```python
from build123d import *

# Parameters (mm, degrees)
F1_DEPTH = 57
F2_DEPTH = 12


with BuildPart() as f1:
    # F0 (on Right) → F1 (new body)
    with BuildSketch(Plane.YZ):
        Polygon((1107.558378, 1620.736191), (1544.042206, 643.137381), (1586.458342, 548.137381), (1690.497414, 548.137381), (1132.390367, 1798.137381), (1064.487016, 1717.203709), align=None)
        Polygon((207.647976, 548.137381), (287.352976, 643.137381), (1107.558378, 1620.736191), (1064.487016, 1717.203709), (83.640367, 548.137381), align=None)
        Polygon((1586.458342, 548.137381), (1544.042206, 643.137381), (287.352976, 643.137381), (207.647976, 548.137381), align=None)
    extrude(amount=-F1_DEPTH)

    # F0 (on Right) → F2 (join)
    with BuildSketch(Plane.YZ):
        Polygon((287.352976, 643.137381), (1544.042206, 643.137381), (1107.558378, 1620.736191), align=None)
    extrude(amount=-F2_DEPTH)


solid = f1.part
```
Geometry: final body of the model. Coordinates: model frame, mm. A direction names the side the tool comes from. Round coordinates to 2 decimals unless told otherwise and drop trailing zeros. Write each loop counter-clockwise with the first axis right and the second up, starting at its lowest first coordinate (ties: lowest second). Pieces come first, ordered by that corner, then holes.
Item 1: Material intervals for L1, parallel to X at y = 1159, z = 869.5; L2, parallel to Y at x = -39.5, z = 964.5; L3, parallel to Y at x = -30.5, z = 651, sorted ascending.
Item 2: Mould query, pull axis Z, two halves, no side actions, for faces 1 (the face through (-28, 876, 548.137)), 2 (the face through (0, 876, 904)), 3 (the face through (-34.185, 1322.745, 1138.78)). Classes: +Z half, -Z half, draft (parallel to the pull), parting line (faces both ways), or undercut.
Item 3: Section query D-D (z = 1667). Return loops of the section in (x, y).
Item 4: Section query B-B (y = 595). Return loops of the section in (x, z), plus the area to 3 significant figures.
Item 5: Set-up query: faces 4 (the face through (-57, 705, 1176)), 5 (the face through (-12, 907, 922)). Return all of +Z, -Z, +X, -X, +Y, -Y with unobstructed straight access to the full face (end or side cutting, diameter ignored); none if empty.
Item 6: Section query C-C (z = 1493). Return loops of the section in (x, y).
Item 7: Section query A-A (x = -27.5). Return loops of the section in (y, z).
Item 8: Pin query (flat end, axial travel): P1, Ø10, axis at x = -48.5, z = 1497.5, coming from the -Y side; P2, Ø2, axis at x = -38.5, y = 680.5, coming from the +Z side; P3, Ø13.5, axis at x = -45, y = 924, coming from the +Z side. Return the tip coordinate at first contact, or that it passes through.
Completed:
1. L1: x = -12 to 0
1. L2: y = 432.97 to 556.98, 1400.56 to 1504.6
1. L3: y = 169.94 to 293.95, 1540.53 to 1644.57
2. face 1: -Z half
2. face 2: draft
2. face 3: undercut
3. outline: (-57, 1022.37) - (0, 1022.37) - (0, 1190.94) - (-57, 1190.94) - close
4. outline: (-57, 548.14) - (0, 548.14) - (0, 1157.62) - (-57, 1157.62) - (-57, 1009.82) - (-12, 1009.82) - (-12, 643.14) - (-57, 643.14) - close
4. area: 18,200 mm2
5. face 4: +Z, -Z, -X, +Y, -Y
5. face 5: -X
6. outline: (-57, 876.38) - (0, 876.38) - (0, 1268.63) - (-57, 1268.63) - (-57, 1164.59) - (-12, 1164.59) - (-12, 1000.39) - (-57, 1000.39) - close
7. outline: (83.64, 548.14) - (1690.5, 548.14) - (1132.39, 1798.14) - close; hole (287.35, 643.14) - (1544.04, 643.14) - (1107.56, 1620.74) - close
8. P1: stops at y = 875.96
8. P2: stops at z = 1260.72
8. P3: stops at z = 1557.8
